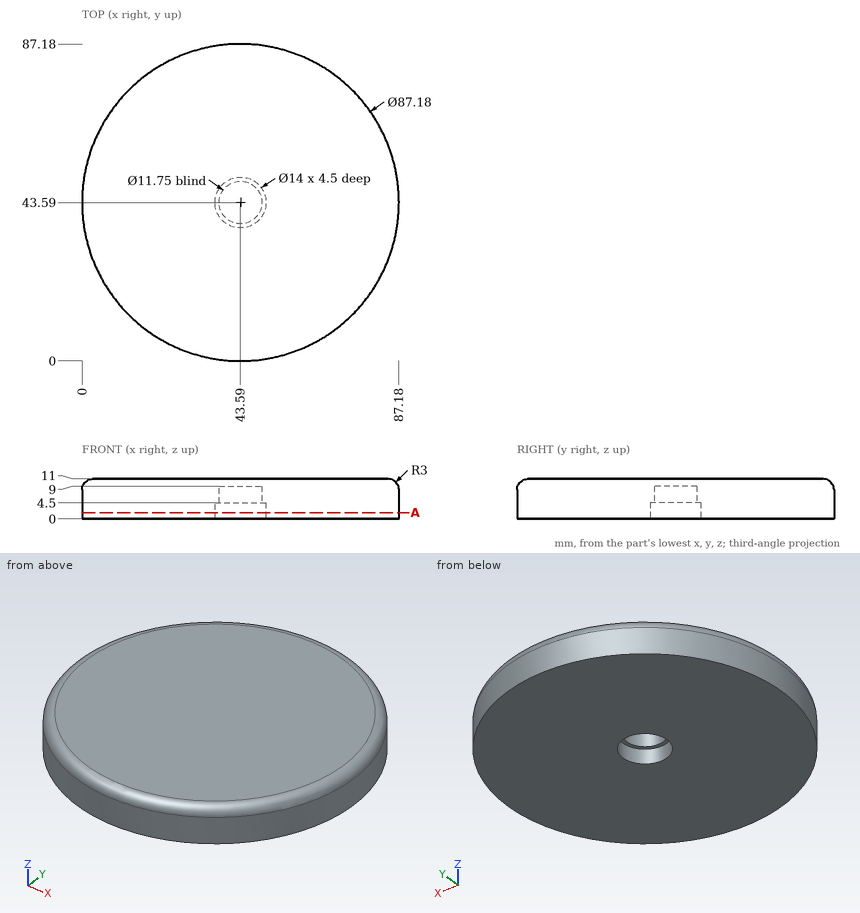
Answer from the drawing. Dimensions are ordinates in mm from the lowest x, y and z of the part. Coordinates: 2 decimals unless noted, no trailing zeros. Write each loop counter-clockwise with the first axis right and the second up, starting at its lowest first coordinate (ties: lowest second). Pieces come first, ordered by that corner, then holes. Notation, with made-up numbers: M 85,-32.75 L 102,-32.75 A15 ccw 102,-26.75 Z; hole C -35.75,15.5 d1. An arc over 180 degrees is marked long. Use one line per item in the form item = value. Start each with the question number.
1. The part is cut by section A-A (z = 1.75). Give the vertices of the cut face in (x, y), plus the area to 3 significant figures.
2. Each of these flat-tipped pins is pushed along its axis until it touches: P1, Ø13, axis at x = 41, y = 41.5, coming from the -Z side; P2, Ø1.5, axis at x = 52, z = 6.5, coming from the +Y side; P3, Ø4, axis at y = 47, z = 1, coming from the +X side; P4, Ø4, axis at x = 41.5, y = 46.5, coming from the -Z side. Where does it stop, or does it pass through?
3. Straight lines are drawn through the part: probe 1 along Y at (x, z) = (45, 1.5); probe 2 along Z at (x, y) = (48, 40); probe 3 along Y at (x, z) = (4, 8.5). For each, find the intervals that lie inside material, in ascending order. Write a range as from..to.
Evaluation:
q1.outline = C 43.59,43.59 d87.18; hole C 43.59,43.59 d14
q1.area = 5,820 mm^2
q2.P1 = 0
q2.P2 = 86.5
q2.P3 = 87.16
q2.P4 = 9
q3.probe_1 = 0.02..36.73, 50.45..87.16
q3.probe_2 = 9..11
q3.probe_3 = 25.45..61.73
